Verification items for the finished model (mm, model axes). Face numbers are marked on the shaded views. A direction names the side the tool comes from. Round coordinates to 2 decimals unless told otherwise and drop trailing zeros. Write each loop counter-clockwise with the first axis right and the second up, starting at its lowest first coordinate (ties: lowest second). Pieces come first, ordered by that corner, then holes. Notation, with made-up numbers: (20.5, 16) - (69.5, 16) arc R25 ccw to (69.5, 32) - close; hole circle Ø5 at (-37.75, 75.25). An arc over 180 degrees is marked (long way). Answer as a JSON object with one key per item and string values.
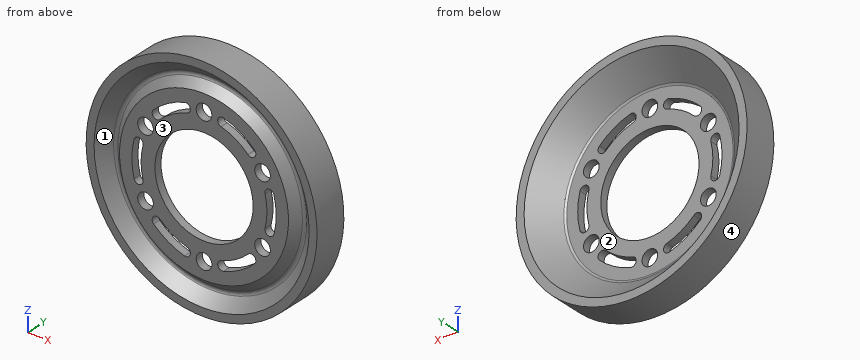
```python
from build123d import *

# Parameters (mm, degrees)
SKETCH1_R           = 37.595
BOSS_EXTRUDE1_DEPTH = 5.5
SKETCH3_R           = 16
SKETCH3_R_2         = 2.55
CUT_EXTRUDE1_DEPTH  = 11
FILLET1_R           = 1
CUT_EXTRUDE2_DEPTH  = 10
CIRPATTERN1_COUNT   = 6


with BuildPart() as part:
    # Sketch1 → Boss-Extrude1 (new, symmetric)
    with BuildSketch(Plane(origin=(0, 0, 0), x_dir=(1, 0, 0), z_dir=(0, 1, 0))):
        with Locations(Location((0, 0, 0), (0, 0, 270))):
            Circle(SKETCH1_R)
    extrude(amount=BOSS_EXTRUDE1_DEPTH, both=True)

    # Sketch2 → Cut-Revolve1 (revolve, cut)
    with BuildSketch(Plane(origin=(0, 0, 0), x_dir=(0, 0, -1), z_dir=(1, 0, 0))):
        Polygon((0, 5.5), (0, -2), (-27.5, -2), (-35, 5.5), align=None)
        Polygon((0, -5.5), (0, -4.5), (-27.5, -4.5), (-30.75, -1.25), (-35, -5.5), align=None)
    revolve(axis=Axis((0, 19.347580659, 0), (0, -1, 0)), mode=Mode.SUBTRACT)

    # Sketch3 → Cut-Extrude1 (cut)
    with BuildSketch(Plane(origin=(0, -2, 0), x_dir=(1, 0, 0), z_dir=(0, 1, 0))):
        with Locations(Location((0, 0, 0), (0, 0, 270))):
            Circle(SKETCH3_R)
        with Locations(Location((0, 22, 0), (0, 0, 270))):
            Circle(SKETCH3_R_2)
        with Locations(Location((19.052558883, 11, 0), (0, 0, 270))):
            Circle(SKETCH3_R_2)
        with Locations(Location((19.052558883, -11, 0), (0, 0, 270))):
            Circle(SKETCH3_R_2)
        with Locations(Location((0, -22, 0), (0, 0, 270))):
            Circle(SKETCH3_R_2)
        with Locations(Location((-19.052558883, -11, 0), (0, 0, 270))):
            Circle(SKETCH3_R_2)
        with Locations(Location((-19.052558883, 11, 0), (0, 0, 270))):
            Circle(SKETCH3_R_2)
    extrude(amount=-CUT_EXTRUDE1_DEPTH, mode=Mode.SUBTRACT)

    # Fillet1
    fillet1_edges = [part.edges().sort_by_distance(p)[0] for p in [
        (0, -1.25, -30.75),
        (0, -2, -27.5),
    ]]
    fillet(fillet1_edges, radius=FILLET1_R)

    # Sketch4 → Cut-Extrude2 (cut)
    with BuildSketch(Plane(origin=(0, -2, 0), x_dir=(1, 0, 0), z_dir=(0, 1, 0))):
        with BuildLine():
            ThreePointArc((-16.420108098, 16.811604625), (-16.445097238, 14.690431472), (-14.323924085, 14.665442332))
            ThreePointArc((-14.323924085, 14.665442332), (-10.25, 17.753520778), (-5.538683575, 19.737603306))
            ThreePointArc((-5.538683575, 19.737603306), (-4.499738229, 21.587087712), (-6.349222635, 22.626033058))
            ThreePointArc((-6.349222635, 22.626033058), (-11.75, 20.351596989), (-16.420108098, 16.811604625))
        make_face()
    cut_extrude2 = extrude(amount=-CUT_EXTRUDE2_DEPTH, mode=Mode.SUBTRACT)

    # CirPattern1: Cut-Extrude2 ×6 about axis
    cirpattern1_axis = Axis((0, 0, 0), (0, 1, 0))
    for i in range(1, CIRPATTERN1_COUNT):
        add(cut_extrude2.rotate(cirpattern1_axis, i * 360 / CIRPATTERN1_COUNT), mode=Mode.SUBTRACT)


solid = part.part
```
1. Material ranges on probe 1 along X at (y, z) = (-3.5, 14.5); probe 2 along X at (y, z) = (-3.05, 11); probe 3 along X at (y, z) = (1.5, 19), recorded low to high. Write a range as from..to.
Completed:
{"probe 1": "x = -34.69..-29.64, -24.54..-16.22, -14.53..-6.76, 6.76..14.53, 16.22..24.54, 29.64..34.69", "probe 2": "x = -35.95..-30.63, -26.78..-21.6, -16.5..-11.62, 11.62..16.5, 21.6..26.78, 30.63..35.95", "probe 3": "x = -32.44..-24.49, 24.49..32.44"}
2. Access from +Z, -Z, +X, -X, +Y, -Y to the whole of each face (thin tool, end or side, straight path). Record for the marked faces 1 and 2.
Completed:
{"face 1": "-Y", "face 2": "+Y"}
3. Cross-section at B-B (x = 0). Count the separate pieces of the cut face and the enclosed holes in it, plus the area to 3 significant figures.
Completed:
{"separate pieces": "4", "enclosed holes": "0", "area": "163 mm^2"}
4. Cross-section at A-A (y = 1.5). Record the boundary of the cut face in (x, z) (3 decimals), plus the area to 3 significant figures.
Completed:
{"outline": "circle Ø75.19 at (0, 0); hole circle Ø62 at (0, 0)", "area": "1,420 mm^2"}
5. Go/stop test with flat-tipped pins: pin 1 (8 mm diameter, centred on x = -19.05, z = 11, fed in from +Y); pin 2 (8 mm diameter, centred on x = 19.05, z = -11, fed in from -Y); pin 3 (5 mm diameter, centred on x = -21.5, y = 0.5, fed in from +Z). Record where each tip stops, or that it passes through.
Completed:
{"pin 1": "stops at y = -2", "pin 2": "stops at y = -4.5", "pin 3": "stops at z = 32.44"}
6. Mould release check, pull along X, two halves, no side actions. Record for the marked faces 3 and 4: released by +X, released by -X, zero draft, split by the parting line, or undercut.
Completed:
{"face 3": "undercut", "face 4": "split by the parting line"}
